The drawing under review shows one solid part. Ordinate dimensions are in mm from its lowest x, y, z. Coordinates: 2 decimals unless noted, no trailing zeros. Write each loop counter-clockwise with the first axis right and the second up, starting at its lowest first coordinate (ties: lowest second). Pieces come first, ordered by that corner, then holes.
1) To check wall thickness, follow line 1 along Z through (x, y) = (8.25, 23.75); line 2 along X through (y, z) = (7.25, 61); line 3 along X through (y, z) = (18.75, 62.5). State the ranges of each line that lie inside material, in increasing order.
2) Insertion check: P1, Ø12, axis at y = 19.5, z = 34.5, coming from the +X side; P2, Ø1.5, axis at x = 7, y = 12, coming from the +Z side; P3, Ø0.9, axis at y = 28.5, z = 61.5, coming from the +X side; P4, Ø8, axis at x = 12, z = 14.5, coming from the -Y side. Each pin has a flat end and moves straight along its axis. Give the tip position at first contact, or say it passes through.
3) We need section C-C on x = 14. Write out the cut boundary in (y, z), then the cut area to 3 significant figures.
4) We need section B-B on z = 15. Write out the cut boundary in (x, y).
5) Mouldability with a two-part tool opening along Y and no side actions: class the marked faces 1, 2, 3 and 4 as pulls with the +Y half, pulls with the -Y half, needs draft (parallel to the pull), parting line crosses it, or undercut.
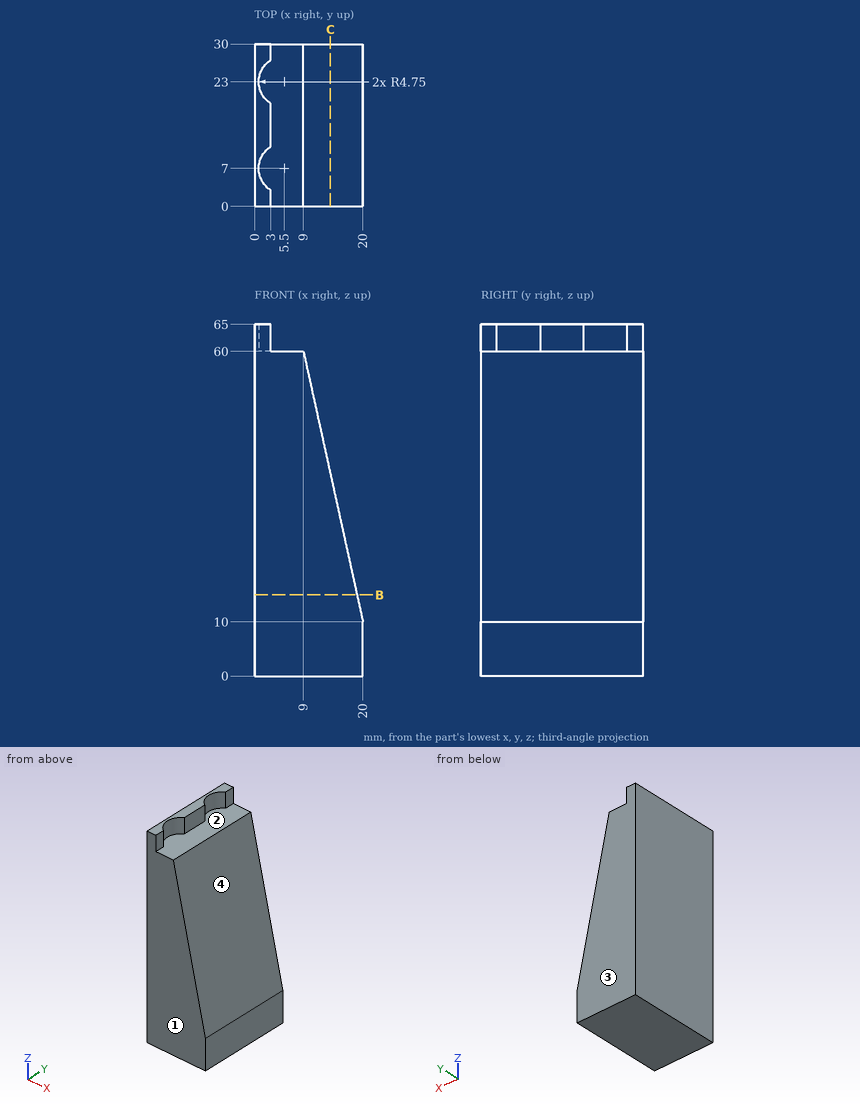
Result:
1. line 1: z = 0 to 60
1. line 2: x = 0 to 0.76
1. line 3: x = 0 to 3
2. P1: stops at x = 15.93
2. P2: stops at z = 60
2. P3: stops at x = 3
2. P4: stops at y = 0
3. outline: (0, 0) - (30, 0) - (30, 37.27) - (0, 37.27) - close
3. area: 1,120 mm2
4. outline: (0, 0) - (18.9, 0) - (18.9, 30) - (0, 30) - close
5. face 1: pulls with the -Y half
5. face 2: undercut
5. face 3: pulls with the +Y half
5. face 4: needs draft
